Check sheet for the modelled part. Datum: model origin and axes. Units: mm. A direction names the side the tool comes from. Coordinates: 2 decimals unless noted, no trailing zeros. Loops run counter-clockwise (first coordinate to the right, second up) from the corner with the lowest first, then second, coordinate; pieces in that order, holes last. Notation, with made-up numbers: M 35.25,57 L 46.25,57 A4 ccw 46.25,64 Z; hole C 68,-1.75 d4. An arc over 180 degrees is marked long. Use CSV: the item, a comma, the result in double quotes. Start each with the question number.
(1) Go/stop test with a flat-tipped pin: pin 1 Ø12 at (x, z) = (125, -16.5) entering from -Y. Record where the tip stops, or that it passes through.
(2) Scan lines: line 1 (Y direction, x = 504.5, z = -7.5); line 2 (Z direction, x = 208.5, y = 16); line 3 (Y direction, x = 41.91, z = -22.9). Record each from-to range of solid material in increasing order.
(3) Section check C-C on x = 355. Record the cut outline in (y, z).
(4) Set-up check for faces 1 (the flat face through (275, 12, 0)), 2 (the flat face through (275, 12, -1.651)): record each of +Z, -Z, +X, -X, +Y, -Y from which the full face is reachable in a straight line by a thin tool's end or side.
(5) Section check B-B on x = 41.91. Record the cut outline in (y, z).
(6) Section check A-A on z = -11.5. Record the cut outline in (x, y), and give its area (3 significant figures).
(7) Draft check along X on faces 3 (the flat face through (0, 1, -12)), 4 (the cylindrical face through (46.634, 13.172, -0.814)), 5 (the flat face through (275, 23.368, -12)). Enter one of: pulls with the +X half, pulls with the -X half, needs draft (parallel to the pull), parting line crosses it, or undercut.
from build123d import *

# Parameters (mm, degrees)
BOSS_EXTRUDE1_DEPTH = 558.8
CUT_EXTRUDE1_REACH  = 561.776
SKETCH3_R           = 4.953


with BuildPart() as part:
    # Sketch2 → Boss-Extrude1 (new body)
    with BuildSketch(Plane(origin=(0, 0, 0), x_dir=(0, 0, -1), z_dir=(1, 0, 0))):
        with BuildLine():
            Line((5.08, 0), (18.288, 0))
            ThreePointArc((18.288, 0), (21.880102448, 1.487897552), (23.368, 5.08))
            Line((23.368, 5.08), (23.368, 18.288))
            ThreePointArc((23.368, 18.288), (21.880102448, 21.880102448), (18.288, 23.368))
            Line((18.288, 23.368), (5.08, 23.368))
            ThreePointArc((5.08, 23.368), (1.487897552, 21.880102448), (0, 18.288))
            Line((0, 18.288), (0, 5.08))
            ThreePointArc((0, 5.08), (1.487897552, 1.487897552), (5.08, 0))
        make_face()
        with BuildLine():
            Line((2.921, 1.651), (20.447, 1.651))
            ThreePointArc((20.447, 1.651), (21.345025612, 2.022974388), (21.717, 2.921))
            Line((21.717, 2.921), (21.717, 20.447))
            ThreePointArc((21.717, 20.447), (21.345025612, 21.345025612), (20.447, 21.717))
            Line((20.447, 21.717), (2.921, 21.717))
            ThreePointArc((2.921, 21.717), (2.022974388, 21.345025612), (1.651, 20.447))
            Line((1.651, 20.447), (1.651, 2.921))
            ThreePointArc((1.651, 2.921), (2.022974388, 2.022974388), (2.921, 1.651))
        make_face(mode=Mode.SUBTRACT)
    extrude(amount=BOSS_EXTRUDE1_DEPTH)

    # Cut-Extrude1: up to this face of the body (flat: up to its plane)
    cut_extrude1_end = Plane(part.part.faces().sort_by_distance((279.4, 11.684, -23.368))[0])
    # Sketch3 → Cut-Extrude1 (cut, up to the picked face)
    with BuildSketch(Plane.XY, mode=Mode.PRIVATE) as cut_extrude1_sk1:
        with Locations((41.91, 11.684)):
            Circle(SKETCH3_R)
    cut_extrude1_tool1 = split(extrude(cut_extrude1_sk1.sketch, amount=-CUT_EXTRUDE1_REACH, mode=Mode.PRIVATE), bisect_by=cut_extrude1_end, keep=Keep.BOTH, mode=Mode.PRIVATE)
    add(cut_extrude1_tool1.solids().sort_by(Axis((41.91, 11.684, 0), (0, 0, -1)))[0], mode=Mode.SUBTRACT)


solid = part.part
Outcome:
1,pin 1,"stops at y = 0"
2,line 1,"y = 0 to 1.65, 21.72 to 23.37"
2,line 2,"z = -23.37 to -21.72, -1.65 to 0"
2,line 3,"y = 2.95 to 6.73, 16.64 to 20.42"
3,outline,"M 0,-18.29 A5.08 ccw 5.08,-23.37 L 18.29,-23.37 A5.08 ccw 23.37,-18.29 L 23.37,-5.08 A5.08 ccw 18.29,0 L 5.08,0 A5.08 ccw 0,-5.08 Z; hole M 1.65,-20.45 A1.27 ccw 2.92,-21.72 L 20.45,-21.72 A1.27 ccw 21.72,-20.45 L 21.72,-2.92 A1.27 ccw 20.45,-1.65 L 2.92,-1.65 A1.27 ccw 1.65,-2.92 Z"
4,face 1,"+Z, +X, -X, +Y, -Y"
4,face 2,"+X, -X"
5,outline,"M 0,-18.29 A5.08 ccw 5.08,-23.37 L 6.73,-23.37 L 6.73,-21.72 L 2.92,-21.72 A1.27 cw 1.65,-20.45 L 1.65,-2.92 A1.27 cw 2.92,-1.65 L 6.73,-1.65 L 6.73,0 L 5.08,0 A5.08 ccw 0,-5.08 Z; M 16.64,-23.37 L 18.29,-23.37 A5.08 ccw 23.37,-18.29 L 23.37,-5.08 A5.08 ccw 18.29,0 L 16.64,0 L 16.64,-1.65 L 20.45,-1.65 A1.27 cw 21.72,-2.92 L 21.72,-20.45 A1.27 cw 20.45,-21.72 L 16.64,-21.72 Z"
6,outline,"M 0,0 L 558.8,0 L 558.8,1.65 L 0,1.65 Z; M 0,21.72 L 558.8,21.72 L 558.8,23.37 L 0,23.37 Z"
6,area,"1,850 mm²"
7,face 3,"pulls with the -X half"
7,face 4,"undercut"
7,face 5,"needs draft"
